Geometry: final body of the model. Coordinates: model frame, mm. Give positions to 0.01 mm unless a question says otherwise; leave off trailing zeros. Loops run counter-clockwise (first coordinate to the right, second up) from the corner with the lowest first, then second, coordinate; pieces in that order, holes last. Notation, with made-up numbers: M -15.5,18 L 21.5,18 A21 cw 21.5,25 Z; hole C 25,68 d5. An arc over 180 degrees is marked long. Put each result on its own line as item: value.
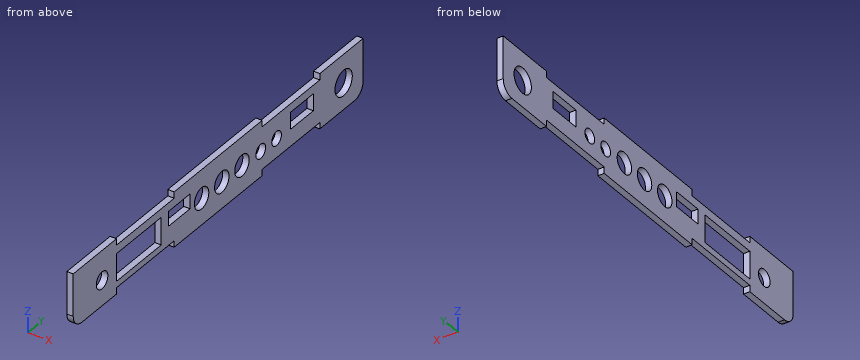
```python
from build123d import *

# Parameters (mm, degrees)
SKETCH_1_W          = 26
SKETCH_1_H          = 201
EXTRUDE_1_DEPTH     = 3
SKETCH_5_W          = 3
SKETCH_5_H          = 40
CUT_EXTRUDE_1_DEPTH = 3
FILLET_1_R          = 6
FILLET_2_R          = 6
SKETCH_6_R          = 4
SKETCH_6_R_2        = 5
SKETCH_6_R_3        = 3.355744506
SKETCH_6_R_4        = 6
SKETCH_6_W          = 13
SKETCH_6_H          = 31
SKETCH_6_W_2        = 7
SKETCH_6_H_2        = 15
SKETCH_6_W_3        = 8
SKETCH_6_H_3        = 16
CUT_EXTRUDE_2_DEPTH = 3


with BuildPart() as part:
    # 草图1 → 凸台-拉伸1 (new body)
    with BuildSketch(Plane(origin=(0, 0, 0), x_dir=(0, 0, -1), z_dir=(1, 0, 0))):
        with Locations((-160.472227767, -5.969447374)):
            Rectangle(SKETCH_1_W, SKETCH_1_H)
    extrude(amount=EXTRUDE_1_DEPTH)

    # 草图5 → 切除-拉伸1 (cut)
    with BuildSketch(Plane(origin=(3, 0, 0), x_dir=(0, 0, -1), z_dir=(1, 0, 0))):
        with Locations((-148.972227767, 44.530552626)):
            Rectangle(SKETCH_5_W, SKETCH_5_H)
        with Locations((-171.972227767, 44.530552626)):
            Rectangle(SKETCH_5_W, SKETCH_5_H)
        with Locations((-171.972227767, -56.469447374)):
            Rectangle(SKETCH_5_W, SKETCH_5_H)
        with Locations((-148.972227767, -56.469447374)):
            Rectangle(SKETCH_5_W, SKETCH_5_H)
    extrude(amount=-CUT_EXTRUDE_1_DEPTH, mode=Mode.SUBTRACT)

    # 圆角1
    fillet_1_edges = [part.edges().sort_by_distance(p)[0] for p in [
        (1.5, 94.530552626, 147.472227767),
    ]]
    fillet(fillet_1_edges, radius=FILLET_1_R)

    # 圆角2
    fillet_2_edges = [part.edges().sort_by_distance(p)[0] for p in [
        (1.5, -106.469447374, 147.472227767),
    ]]
    fillet(fillet_2_edges, radius=FILLET_2_R)

    # 草图6 → 切除-拉伸2 (cut)
    with BuildSketch(Plane.ZY):
        with Locations((159.472227767, -86.469447374)):
            Circle(SKETCH_6_R)
        with Locations((159.972227767, -17.469447374)):
            Circle(SKETCH_6_R_2)
        with Locations((159.972227767, -3.469447374)):
            Circle(SKETCH_6_R_2)
        with Locations((159.972227767, 10.530552626)):
            Circle(SKETCH_6_R_2)
        with Locations((159.472227767, 23.530552626)):
            Circle(SKETCH_6_R_3)
        with Locations((159.472227767, 34.530552626)):
            Circle(SKETCH_6_R_3)
        with Locations((159.972227767, 81.030552626)):
            Circle(SKETCH_6_R_4)
        with Locations((159.972227767, -60.969447374)):
            Rectangle(SKETCH_6_W, SKETCH_6_H)
        with Locations((162.972227767, -32.969447374)):
            Rectangle(SKETCH_6_W_2, SKETCH_6_H_2)
        with Locations((162.472227767, 52.030552626)):
            Rectangle(SKETCH_6_W_3, SKETCH_6_H_3)
    extrude(amount=-CUT_EXTRUDE_2_DEPTH, mode=Mode.SUBTRACT)


solid = part.part
```
Item 1: Pin query (flat end, axial travel): pin 1 Ø2 at (y, z) = (-77, 156.5) entering from -X; pin 2 Ø0.9 at (x, y) = (1.5, -61) entering from -Z; pin 3 Ø0.9 at (x, z) = (2, 148) entering from -Y. Return the tip coordinate at first contact, or that it passes through.
Output values:
pin 1: x = 0
pin 2: z = 150.47
pin 3: y = -103.75
Item 2: Section A-A on y = -51. Output: boundary loops of the cut face in (x, z).
Output values:
outline: M 0,150.47 L 3,150.47 L 3,153.47 L 0,153.47 Z; M 0,166.47 L 3,166.47 L 3,170.47 L 0,170.47 Z
Item 3: Line query: probe 1 along Y at (x, z) = (1.8, 171.75); probe 2 along Y at (x, z) = (1.2, 153.75); probe 3 along Z at (x, y) = (2.85, -73.5). Output: solid intervals per line, ascending. Write a range as [from, to].
Output values:
probe 1: [-106.47, -76.47], [-36.47, 24.53], [64.53, 94.53]
probe 2: [-106.47, -76.47], [-45.47, 94.53]
probe 3: [150.47, 153.47], [166.47, 170.47]
Item 4: Section C-C on y = 41. Output: boundary loops of the cut face in (x, z).
Output values:
outline: M 0,150.47 L 3,150.47 L 3,170.47 L 0,170.47 Z
Item 5: Section B-B on x = 1.5. Count the separate pieces of the cut face and the enclosed holes in it, then the cut area to 3 significant figures.
Output values:
separate pieces: 1
enclosed holes: 10
area: 3,620 mm²
